Verification items for this drawing (mm, ordinates from the low corner). Round coordinates to 2 decimals unless told otherwise and drop trailing zeros. Write each loop counter-clockwise with the first axis right and the second up, starting at its lowest first coordinate (ties: lowest second). Pieces come first, ordered by that corner, then holes. Notation, with made-up numbers: (68, 81) -> (117, 81) arc R8 cw to (117, 94) -> close; hole circle Ø11 at (28, -12.75). An arc over 180 degrees is marked (long way). Put each result on its own line as item: value. Start each with the question number.
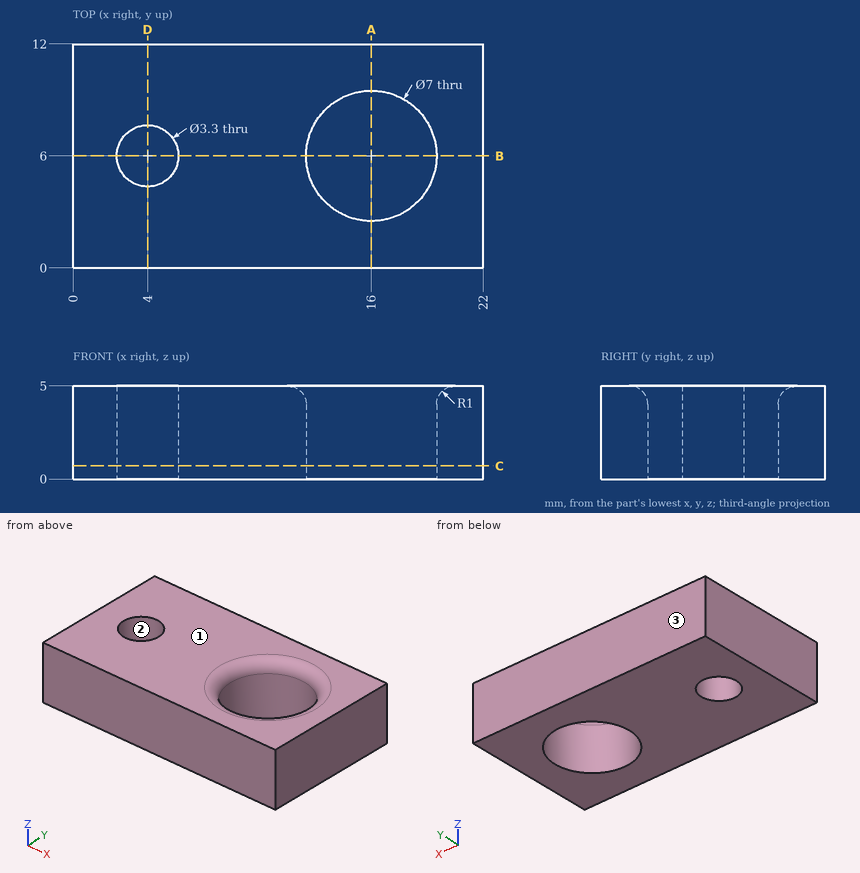
1. Section check A-A, the plane x = 16. Enter the section's corners in (y, z).
2. Section check C-C, the plane z = 0.7. Enter the section's corners in (x, y).
3. Gauge pin test, flat end, axial feed: P1, Ø3, axis at x = 4, y = 6, coming from the -Z side. Record the tip position at first contact, or that the pin passes through.
4. Section check D-D, the plane x = 4. Enter the section's corners in (y, z).
5. Draft check along Y on the marked faces 1, 2 and 3. Enter one of: released by +Y, released by -Y, zero draft, split by the parting line, or undercut.
6. Section check B-B, the plane y = 6. Enter the section's corners in (x, z).
7. Material ranges on L1, parallel to X at y = 7.5, z = 3.4; L2, parallel to Y at x = 16, z = 2.4; L3, parallel to X at y = 8.5, z = 4.45, recorded low to high. Write a range as [from, to].
Reply:
1. outline: (0, 0) -> (2.5, 0) -> (2.5, 4) arc R1 ccw to (1.5, 5) -> (0, 5) -> close; (9.5, 0) -> (12, 0) -> (12, 5) -> (10.5, 5) arc R1 ccw to (9.5, 4) -> close
2. outline: (0, 0) -> (22, 0) -> (22, 12) -> (0, 12) -> close; hole circle Ø3.3 at (4, 6); hole circle Ø7 at (16, 6)
3. P1: passes through
4. outline: (0, 0) -> (4.35, 0) -> (4.35, 5) -> (0, 5) -> close; (7.65, 0) -> (12, 0) -> (12, 5) -> (7.65, 5) -> close
5. face 1: zero draft
5. face 2: undercut
5. face 3: released by +Y
6. outline: (0, 0) -> (2.35, 0) -> (2.35, 5) -> (0, 5) -> close; (5.65, 0) -> (12.5, 0) -> (12.5, 4) arc R1 ccw to (11.5, 5) -> (5.65, 5) -> close; (19.5, 0) -> (22, 0) -> (22, 5) -> (20.5, 5) arc R1 ccw to (19.5, 4) -> close
7. L1: x = [0, 3.31], [4.69, 12.84], [19.16, 22]
7. L2: y = [0, 2.5], [9.5, 12]
7. L3: x = [0, 13.4], [18.6, 22]
